Could you check a few things on this model? Use its own coordinates, in mm. A direction names the side the tool comes from. Give positions to 0.01 mm unless a question says otherwise; leave off trailing zeros. Loops run counter-clockwise (first coordinate to the right, second up) from the corner with the lowest first, then second, coordinate; pieces in that order, holes last. Notation, with made-up numbers: (64.25, 40) -> (86.25, 40) arc R13 ccw to (86.25, 65) -> close; hole circle Ø9 at (-27.75, 62.25). An arc over 180 degrees is marked (long way). Put each result on its own line as item: value.
```python
from build123d import *

# Parameters (mm, degrees)
BOSS_EXTRUDE1_DEPTH = 39
SHELL1_T            = -3
SKETCH2_W           = 33
SKETCH2_H           = 14
CUT_EXTRUDE1_DEPTH  = 730.858236947
SKETCH3_R           = 2.5
CUT_EXTRUDE2_DEPTH  = 504.042108716


with BuildPart() as part:
    # Sketch1 → Boss-Extrude1 (new body)
    with BuildSketch(Plane.XY):
        with BuildLine():
            Line((385.962547752, -201.25), (-287.036202121, -201.25))
            Line((-287.036202121, -201.25), (-308.458422222, -216.25))
            Line((-308.458422222, -216.25), (-308.458422222, -221.25))
            Line((-308.458422222, -221.25), (385.962547752, -221.25))
            ThreePointArc((385.962547752, -221.25), (450.087547752, -157.125), (385.962547752, -93))
            Line((385.962547752, -93), (129, -93))
            ThreePointArc((129, -93), (119, -103), (129, -113))
            Line((129, -113), (385.962547752, -113))
            ThreePointArc((385.962547752, -113), (430.087547752, -157.125), (385.962547752, -201.25))
        make_face()
    extrude(amount=BOSS_EXTRUDE1_DEPTH)

    # Shell1
    shell1_openings = [part.faces().sort_by_distance(p)[0] for p in [
        (-297.747312172, -208.75, 19.5),
    ]]
    offset(amount=SHELL1_T, openings=shell1_openings, kind=Kind.INTERSECTION)

    # Sketch2 → Cut-Extrude1 (cut, through all)
    with BuildSketch(Plane.ZY.offset(-385.962547752)):
        with Locations((19.5, -103)):
            Rectangle(SKETCH2_W, SKETCH2_H)
        with Locations((19.5, -211.25)):
            Rectangle(SKETCH2_W, SKETCH2_H)
    extrude(amount=CUT_EXTRUDE1_DEPTH, mode=Mode.SUBTRACT)

    # Sketch3 → Cut-Extrude2 (cut, through all)
    with BuildSketch(Plane.XY.offset(39)):
        with Locations((129, -103)):
            Circle(SKETCH3_R)
    extrude(amount=-CUT_EXTRUDE2_DEPTH, mode=Mode.SUBTRACT)


solid = part.part
```
1. Thinking about a two-plate mould opening in Y: for faces 4 (the face through (153, -209, 39)), 5 (the face through (259, -93, 19)), 6 (the face through (155, -207, 3)), 7 (the face through (256, -96, 19)), which applies, pulls with the +Y half, pulls with the -Y half, needs draft (parallel to the pull), parting line crosses it, or undercut?
Recorded:
face 4: needs draft
face 5: pulls with the +Y half
face 6: undercut
face 7: undercut
2. I'm going to push flat-ended pins straight in: pin 1 (11.5 mm diameter, centred on x = -116.5, z = 20, fed in from +Y); pin 2 (4 mm diameter, centred on y = -149.5, z = 20, fed in from +X); pin 3 (12 mm diameter, centred on y = -206.5, z = 4.5, fed in from +X). Where does each tip first touch, or does it pass through?
Recorded:
pin 1: stops at y = -201.25
pin 2: stops at x = 449.84
pin 3: stops at x = 433.19
3. If we section it at C-C (x = 17.5): List the corners of the cut face in (y, z) for me.
Recorded:
outline: (-221.25, 0) -> (-201.25, 0) -> (-201.25, 39) -> (-221.25, 39) -> close; hole (-218.25, 3) -> (-204.25, 3) -> (-204.25, 36) -> (-218.25, 36) -> close
4. For faces 1 (the face through (256, -110, 19)), 2 (the face through (447.073, -158.469, 19.269)), 3 (the face through (256, -113, 19)), which set-ups out of +Z, -Z, +X, -X, +Y, -Y let a thin tool reach every point of the face, with its end or its side?
Recorded:
face 1: -X
face 2: none
face 3: +Z, -Z, -X
5. If we section it at A-A (x = 281): List the corners of the cut face in (y, z) for me, then the cut area to 3 significant figures.
Recorded:
outline: (-221.25, 0) -> (-201.25, 0) -> (-201.25, 39) -> (-221.25, 39) -> close; (-113, 0) -> (-93, 0) -> (-93, 39) -> (-113, 39) -> close; hole (-218.25, 3) -> (-204.25, 3) -> (-204.25, 36) -> (-218.25, 36) -> close; hole (-110, 3) -> (-96, 3) -> (-96, 36) -> (-110, 36) -> close
area: 636 mm^2
6. I need wall thicknesses on line 1 (Y direction, x = 129, z = 0.7); line 2 (Y direction, x = 243, z = 28.5); line 3 (Y direction, x = 109, z = 19.5). Which ranges of each line are inside material? Lowest first, please.
Recorded:
line 1: y = -221.25 to -201.25, -113 to -105.5, -100.5 to -93
line 2: y = -221.25 to -218.25, -204.25 to -201.25, -113 to -110, -96 to -93
line 3: y = -221.25 to -218.25, -204.25 to -201.25
7. If we section it at B-B (z = 17): List the corners of the cut face in (x, y) for me (3 decimals).
Recorded:
outline: (-308.458, -221.25) -> (385.963, -221.25) arc R64.125 ccw to (385.963, -93) -> (129, -93) arc R10 ccw to (121.859, -96) -> (385.963, -96) arc R61.125 cw to (385.963, -218.25) -> (-308.458, -218.25) -> close; (-291.321, -204.25) -> (385.963, -204.25) arc R47.125 ccw to (385.963, -110) -> (121.859, -110) arc R10 ccw to (129, -113) -> (385.963, -113) arc R44.125 cw to (385.963, -201.25) -> (-287.036, -201.25) -> close
8. If we section it at D-D (y = -162.5): List the corners of the cut face in (x, z) for me, then the cut area to 3 significant figures.
Recorded:
outline: (429.76, 0) -> (449.86, 0) -> (449.86, 39) -> (429.76, 39) -> close; hole (432.78, 3) -> (446.85, 3) -> (446.85, 36) -> (432.78, 36) -> close
area: 320 mm^2
